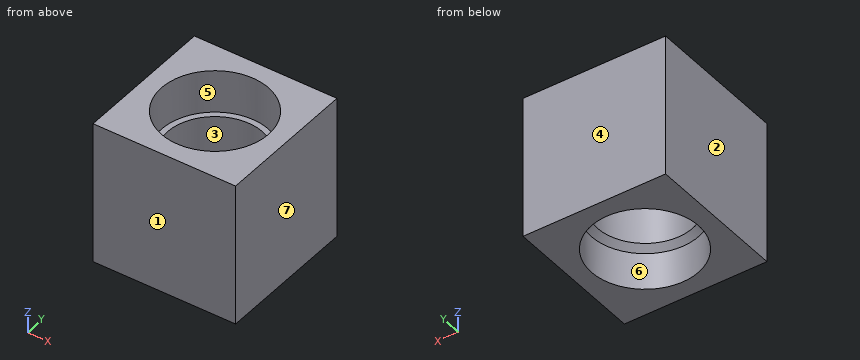
Autodesk Inventor part; units mm, degrees
ref_plane "Work Plane1" through (0, 0, 21) normal (0, 0, 1) x (1, 0, 0)
ref_plane "Work Plane2" through (0, 0, 9) normal (0, 0, -1) x (-1, 0, 0)
ref_plane "YZ Plane" through (0, 0, 0) normal (1, 0, 0) x (0, 1, 0)
sketch "Sketch1" plane through (0, 0, 0) normal (0, 0, 1) x (1, 0, 0)
  circle A0 centre (0, 0) radius 11.25
  line L0 (-15, -15) -> (15, -15)
  line L1 (15, -15) -> (15, 15)
  line L2 (15, 15) -> (-15, 15)
  line L3 (-15, 15) -> (-15, -15)
  point P0 (-15, 0)
  point P1 (0, 15)
  dimension "d0" = 22.5
  dimension "d1" = 30
extrude "Extrusion1" add sketch "Sketch1" along normal blind 30
ref_plane "Work Plane1" through (0, 0, 21) normal (0, 0, 1) x (1, 0, 0)
ref_plane "Work Plane2" through (0, 0, 9) normal (0, 0, -1) x (-1, 0, 0)
sketch "Sketch2" plane through (0, 0, 21) normal (0, 0, 1) x (1, 0, 0)
  circle A0 centre (0, 0) radius 10
  circle A1 centre (0, 0) radius 11.25
  dimension "d6" = 20
extrude "Extrusion2" add sketch "Sketch2" against normal up to surface (12 mm away)
sketch "Sketch3" plane through (0, 0, 0) normal (1, 0, 0) x (0, 1, 0)
  line L0 (15, 30) -> (15, 0)
  line L1 (15, 0) -> (11.25, 0)
  line L2 (11.25, 0) -> (11.25, 9)
  line L3 (11.25, 9) -> (10, 9)
  line L4 (10, 9) -> (10, 21)
  line L5 (10, 21) -> (11.25, 21)
  line L6 (11.25, 21) -> (11.25, 30)
  line L7 (11.25, 30) -> (15, 30)
  line L8 (-15, 0) -> (-15, 30)
  line L9 (-15, 30) -> (-11.25, 30)
  line L10 (-11.25, 30) -> (-11.25, 21)
  line L11 (-11.25, 21) -> (-10, 21)
  line L12 (-10, 21) -> (-10, 9)
  line L13 (-10, 9) -> (-11.25, 9)
  line L14 (-11.25, 9) -> (-11.25, 0)
  line L15 (-11.25, 0) -> (-15, 0)
  line L16 (-10, 9) -> (-11.25, 7.75)
  line L17 (0, -4) -> (0, 24)
  point P0 (0, 0)
  dimension "d9" = 45
revolve "Revolution1" add sketch "Sketch3" angle 360 about axis through (0, 0, -10) along (0, 0, 1) contours L14 L13 L16
equation "\"d0\" = od + hole_oversize"
equation "\"d6\" = damax"
equation "\"id\" = 8"
equation "\"od\" = 22"
equation "\"hole_oversize\" = 0.5"
equation "\"post_oversize\" = 0"
equation "\"bearing_width\" = 9"
equation "\"d4\" = -bearing_width"
equation "\"d5\" = -bearing_width"
equation "\"damax\" = 20"
properties part number "pinch_wheel_hobbing_jig"
For this review, take the finished solid that the model builds, in its own axes (mm). Face numbers are marked on the shaded views. A direction names the side the tool comes from. Round coordinates to 2 decimals unless told otherwise and drop trailing zeros. Write each loop counter-clockwise with the first axis right and the second up, starting at its lowest first coordinate (ties: lowest second). Pieces come first, ordered by that corner, then holes. Notation, with made-up numbers: M -0.5,0.5 L 34.5,0.5 A32 ccw 34.5,39.5 Z; hole C -8.5,13 d11. An arc over 180 degrees is marked long. One line per item, written item: value. Start each with the question number.
(1) We need section C-C (z = 3.5). Give the boundary of the cut face in (x, y).
(2) We need section A-A (y = 0). Give the boundary of the cut face in (x, z).
(3) The part is to be moulded in two halves that separate along Y. For the marked faces 1, 2, 3 and 4, say which applies: released by +Y, released by -Y, zero draft, split by the parting line, or undercut.
(4) Wall thickness on line 1 (X direction, y = 0, z = 6.25); line 2 (Y direction, x = 0, z = 16.5): over which ranges is each line inside the solid? List them lowest first.
(5) Machinability: for the marked faces 5, 6 and 7, which of the approach directions +Z, -Z, +X, -X, +Y, -Y give a long, thin tool a straight path to every point of the face, cutting with its end or side? Answer none if there is none.
(6) Insertion check: pin 1 (2 mm diameter, centred on x = 2, y = -9.5, fed in from -Z); pin 2 (16 mm diameter, centred on x = 0, y = 0, fed in from -Z). Each pin has a flat end and moves straight along its axis. Give the tip position at first contact, or say it passes through.
Result:
1. outline: M -15,-15 L 15,-15 L 15,15 L -15,15 Z; hole C 0,0 d22.5
2. outline: M -15,0 L -11.25,0 L -11.25,7.75 L -10,9 L -10,21 L -11.25,21 L -11.25,30 L -15,30 Z; M 10,9 L 11.25,7.75 L 11.25,0 L 15,0 L 15,30 L 11.25,30 L 11.25,21 L 10,21 Z
3. face 1: released by -Y
3. face 2: zero draft
3. face 3: undercut
3. face 4: released by +Y
4. line 1: -15 to -11.25, 11.25 to 15
4. line 2: -15 to -10, 10 to 15
5. face 5: +Z
5. face 6: -Z
5. face 7: +Z, -Z, +X, +Y, -Y
6. pin 1: z = 8.29
6. pin 2: through
